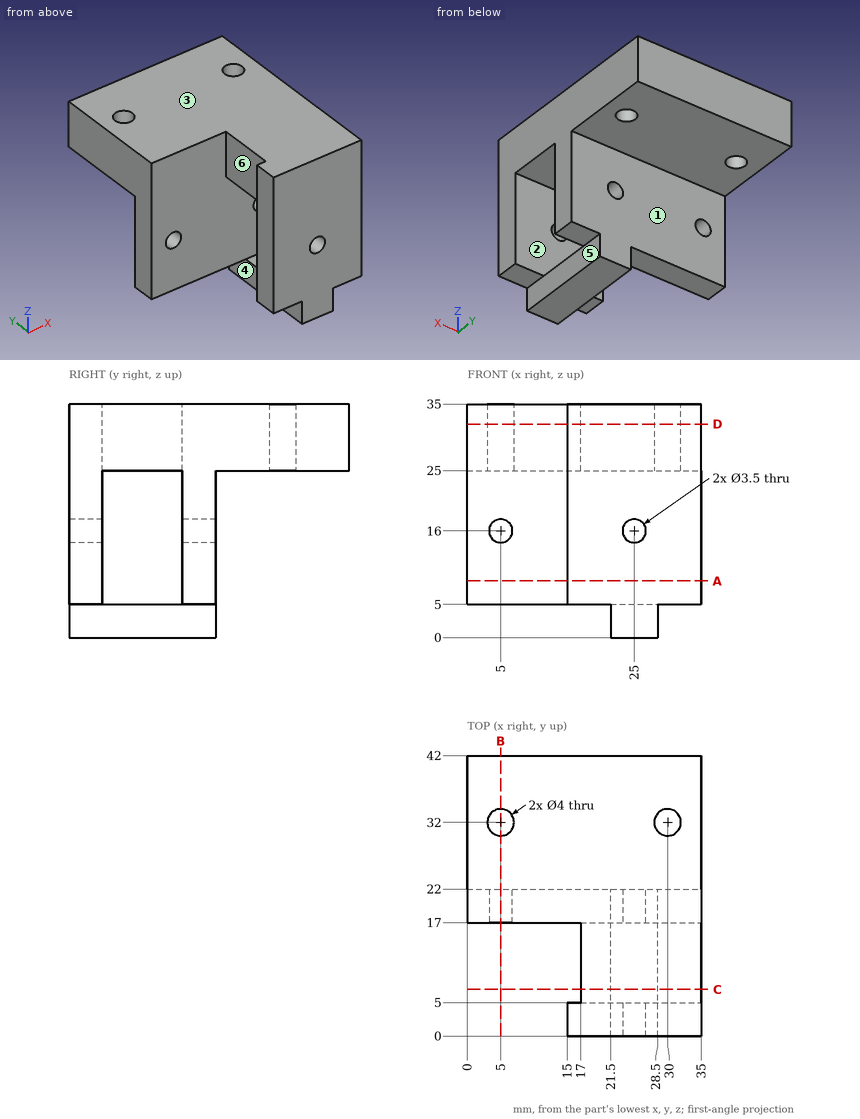
Input: dimensioned drawing with shaded views. Units: mm. Origin: part minimum x, y, z. A direction names the side the tool comes from. Coordinates: 2 decimals unless noted, no trailing zeros. Order: outer loops, then holes, each group sorted by start corner. A loop starts at its lowest first (then second) coordinate and runs counter-clockwise, first axis right, second up. Notation, with made-up numbers: (57, 79) - (96, 79) arc R13 ccw to (96, 103) - close; hole circle Ø1 at (5, -11). An arc over 180 degrees is marked (long way). Return JSON: item names as keys, results as strings. Group by question number.
1. Cut plane D-D (z = 32). Output: boundary loops of the cut face in (x, y), plus the area to 3 significant figures.
2. Cut plane B-B (x = 5). Output: boundary loops of the cut face in (y, z), plus the area to 4 significant figures.
3. Set-up query: the marked faces 4, 5 and 6. Return all of +Z, -Z, +X, -X, +Y, -Y with unobstructed straight access to the full face (end or side cutting, diameter ignored); none if empty.
4. Pin query (flat end, axial travel): pin 1 (12.5 mm diameter, centred on x = 12.5, z = 7, fed in from +Y); pin 2 (3 mm diameter, centred on x = 5, y = 32, fed in from +Z); pin 3 (1.5 mm diameter, centred on x = 11.5, y = 19.5, fed in from -Z); pin 4 (4 mm diameter, centred on y = 1.5, z = 26, fed in from -X). Return the tip coordinate at first contact, or that it passes through.
5. Material intervals for line 1 along Y through (x, z) = (30, 21); line 2 along Y through (x, z) = (5, 32); line 3 along Z through (x, y) = (25, 18.15), sorted ascending. Write a range as [from, to].
6. Cut plane A-A (z = 8.5). Output: boundary loops of the cut face in (x, y), plus the area to 3 significant figures.
7. Pull-direction query (Y, two-part tool) for the marked faces 1, 2 and 3; classes: pulls with the +Y half, pulls with the -Y half, needs draft (parallel to the pull), parting line crosses it, or undercut.
8. Cut plane C-C (y = 7). Output: boundary loops of the cut face in (x, z), plus the area to 3 significant figures.
Resolved:
{
 "1": {"outline": "(0, 17) - (17, 17) - (17, 5) - (15, 5) - (15, 0) - (35, 0) - (35, 42) - (0, 42) - close; hole circle Ø4 at (5, 32); hole circle Ø4 at (30, 32)", "area": "1,170 mm²"},
 "2": {"outline": "(17, 5) - (22, 5) - (22, 14.25) - (17, 14.25) - close; (17, 17.75) - (22, 17.75) - (22, 25) - (30, 25) - (30, 35) - (17, 35) - close; (34, 25) - (42, 25) - (42, 35) - (34, 35) - close", "area": "292.5 mm²"},
 "3": {"face 4": "-Z, -X, +Y, -Y", "face 5": "-Z, +X, +Y, -Y", "face 6": "+Z, -Z, -X"},
 "4": {"pin 1": "stops at y = 22", "pin 2": "passes through", "pin 3": "stops at z = 5", "pin 4": "stops at x = 15"},
 "5": {"line 1": "y = [0, 5], [17, 22]", "line 2": "y = [17, 30], [34, 42]", "line 3": "z = [0, 14.25], [17.75, 35]"},
 "6": {"outline": "(0, 17) - (35, 17) - (35, 22) - (0, 22) - close; (15, 0) - (35, 0) - (35, 5) - (15, 5) - close", "area": "275 mm²"},
 "7": {"face 1": "pulls with the +Y half", "face 2": "undercut", "face 3": "needs draft"},
 "8": {"outline": "(17, 25) - (35, 25) - (35, 35) - (17, 35) - close; (21.5, 0) - (28.5, 0) - (28.5, 5) - (21.5, 5) - close", "area": "215 mm²"}
}
